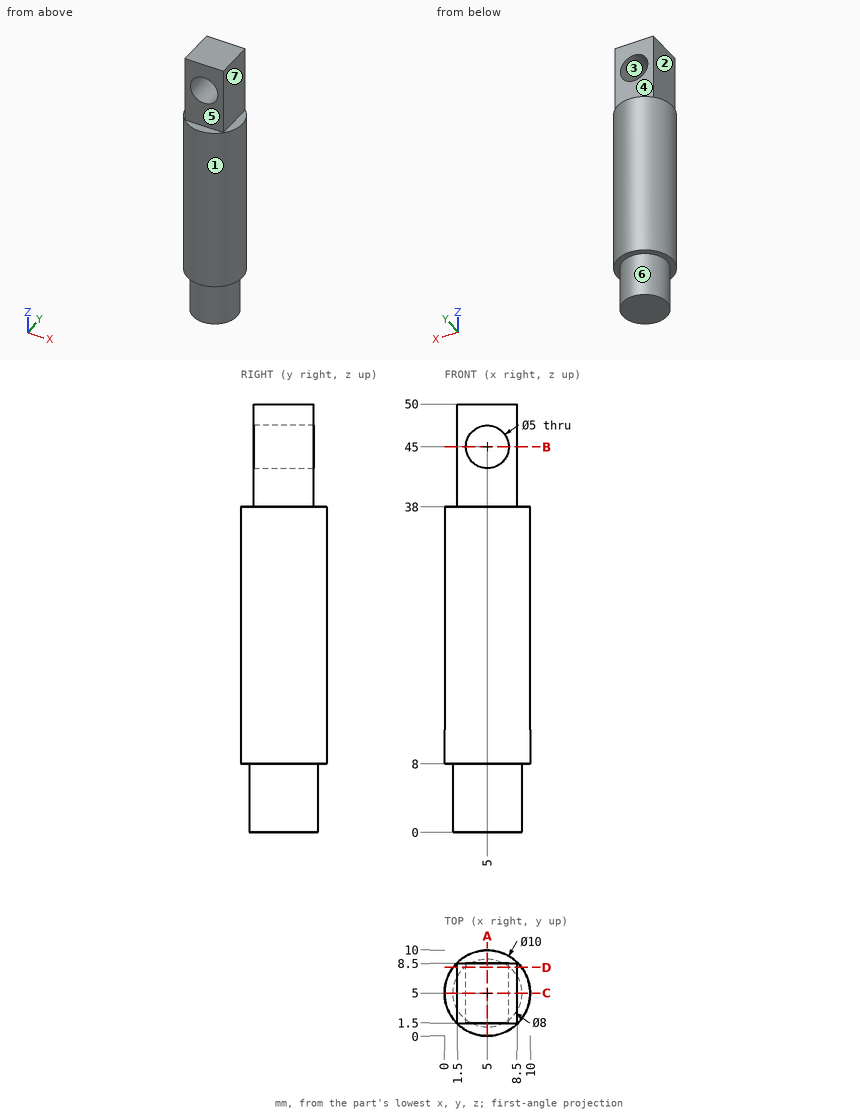
Check sheet for the drawn part. Datum: minimum x, y, z corner. Units: mm. A direction names the side the tool comes from. Round coordinates to 2 decimals unless told otherwise and drop trailing zeros. Loops run counter-clockwise (first coordinate to the right, second up) from the corner with the lowest first, then second, coordinate; pieces in that order, holes last. Notation, with made-up numbers: M -5,23.5 L 38,23.5 A22 cw 38,57.5 Z; hole C 4,-19 d7. An arc over 180 degrees is marked long. One line per question, with ' | ' between items. Start each with the question number.
Item 1: Set-up check for the marked faces 4, 5, 6 and 7: record each of +Z, -Z, +X, -X, +Y, -Y from which the full face is reachable in a straight line by a thin tool's end or side.
Item 2: Scan lines: probe 1 along X at (y, z) = (6.75, 45); probe 2 along Z at (x, y) = (6.5, 0.75); probe 3 along X at (y, z) = (8, 22). Record each from-to range of solid material in increasing order.
Item 3: Gauge pin test, flat ends, axial feed: pin 1 Ø1.5 at (y, z) = (3, 31.5) entering from +X; pin 2 Ø5.5 at (x, z) = (4, 44.5) entering from -Y; pin 3 Ø2 at (x, z) = (5.5, 5.5) entering from +Y. Record the tip position at first contact, or that the pin passes through.
Item 4: Release check for a two-part mould opening along X. For the marked faces 1, 2 and 3 record: released by +X, released by -X, zero draft, split by the parting line, or undercut.
Item 5: Section check C-C (y = 5). Record the boundary of the cut face in (x, z), and give its area (3 significant figures).
Item 6: Section check D-D (y = 8). Record the boundary of the cut face in (x, z), and give its area (3 significant figures).
Item 7: Section check B-B (z = 45). Record the boundary of the cut face in (x, y), and give its area (3 significant figures).
Item 8: Section check A-A (x = 5). Record the boundary of the cut face in (y, z), and give its area (3 significant figures).
Worked out:
1) face 4: +Z, +X, -X, +Y | face 5: +Z, +X, -X, -Y | face 6: -Z | face 7: +Z, +X, +Y, -Y
2) probe 1: 1.5 to 2.5, 7.5 to 8.5 | probe 2: 8 to 38 | probe 3: 1 to 9
3) pin 1: x = 9.84 | pin 2: y = 1.5 | pin 3: y = 9
4) face 1: split by the parting line | face 2: released by -X | face 3: undercut
5) outline: M 0,8 L 1,8 L 1,0 L 9,0 L 9,8 L 10,8 L 10,38 L 8.5,38 L 8.5,50 L 1.5,50 L 1.5,38 L 0,38 Z; hole C 5,45 d5 | area: 428 mm^2
6) outline: M 1,8 L 2.35,8 L 2.35,0 L 7.65,0 L 7.65,8 L 9,8 L 9,38 L 8.5,38 L 8.5,50 L 1.5,50 L 1.5,38 L 1,38 Z; hole C 5,45 d5 | area: 347 mm^2
7) outline: M 1.5,1.5 L 2.5,1.5 L 2.5,8.5 L 1.5,8.5 Z; M 7.5,1.5 L 8.5,1.5 L 8.5,8.5 L 7.5,8.5 Z | area: 14.0 mm^2
8) outline: M 0,8 L 1,8 L 1,0 L 9,0 L 9,8 L 10,8 L 10,38 L 8.5,38 L 8.5,42.5 L 1.5,42.5 L 1.5,38 L 0,38 Z; M 1.5,47.5 L 8.5,47.5 L 8.5,50 L 1.5,50 Z | area: 413 mm^2
